```python
from build123d import *

# Parameters (mm, degrees)
SKETCH_R     = 6
PAD_DEPTH    = 9
SKETCH001_R  = 3
POCKET_DEPTH = 18.001


with BuildPart() as part:
    # Sketch → Pad (new body, symmetric)
    with BuildSketch(Plane.YZ):
        with BuildLine():
            ThreePointArc((83.569101, 625.179701), (-35.530366, 668.105579), (-91.532178, 554.56655))
            ThreePointArc((-170, 0), (-72.883506, 269.093239), (-91.532178, 554.56655))
            Line((-170, 0), (170, 0))
            ThreePointArc((170, 0), (183.382066, 320.41444), (83.569101, 625.179701))
        make_face()
        with Locations((0, 580)):
            Circle(SKETCH_R, mode=Mode.SUBTRACT)
    extrude(amount=PAD_DEPTH, both=True)

    # Sketch001 (on Face7 of Pad) → Pocket (cut, through all)
    with BuildSketch(Plane.YZ.offset(9)):
        with Locations((-53.033009, 526.966991)):
            Circle(SKETCH001_R)
        with Locations((53.033009, 526.966991)):
            Circle(SKETCH001_R)
    extrude(amount=-POCKET_DEPTH, mode=Mode.SUBTRACT)


solid = part.part
```
Work out the finished part from the listing and answer in its coordinate system (mm). Round coordinates to 2 decimals unless told otherwise and drop trailing zeros. Write each loop counter-clockwise with the first axis right and the second up, starting at its lowest first coordinate (ties: lowest second). Pieces come first, ordered by that corner, then holes. Notation, with made-up numbers: (-29.5, 3.25) -> (-21.5, 3.25) arc R15 ccw to (-21.5, 10.25) -> close; hole circle Ø2 at (2, -33.5). An arc over 180 degrees is marked (long way). Write each question's results on one line, items separated by ' | '.
1) The part is cut by section A-A (x = 0.25). Write down the section's boundary in (y, z).
Findings:
outline: (-170, 0) -> (170, 0) arc R900 ccw to (83.57, 625.18) arc R95 ccw to (-91.53, 554.57) arc R700 cw to start; hole circle Ø6 at (-53.03, 526.97); hole circle Ø12 at (0, 580); hole circle Ø6 at (53.03, 526.97)
2) The part is cut by section B-B (y = 97). Write down the section's boundary in (x, z).
Findings:
outline: (-9, 0) -> (9, 0) -> (9, 599.35) -> (-9, 599.35) -> close
3) The part is cut by section C-C (z = 175). Write down the section's boundary in (x, y).
Findings:
outline: (-9, -92.87) -> (9, -92.87) -> (9, 191.59) -> (-9, 191.59) -> close
4) Consider line 1 along Y through (x, z) = (-3.5, 580); line 2 along Z through (x, y) = (-2.75, -11); line 3 along Y through (x, z) = (-4, 568.5). Determine where each line is inside the solid, lowest interval first. Write a range as [from, to].
Findings:
line 1: y = [-95, -6], [6, 106.38] | line 2: z = [0, 674.36] | line 3: y = [-94.3, 111.68]
5) Flat-ended cylindrical pins translate along their axes: pin 1 (10 mm diameter, centred on x = 1, z = 524.5, fed in from +Y); pin 2 (5 mm diameter, centred on x = 0, z = 163.5, fed in from -Y); pin 3 (10 mm diameter, centred on x = 1.5, z = 593, fed in from +Y). Find the tip coordinate at first contact, or state that the pin passes through.
Findings:
pin 1: stops at y = 132.16 | pin 2: stops at y = -97.03 | pin 3: stops at y = 102.57
6) For a pull along Z with two mould halves and no side action, classify faces 1 (the flat face through (9, 49, 267)), 2 (the flat face through (0, -2, 0)), 3 (the cylindrical face through (-0.13, -0.78, 585.95)) as +Z half, -Z half, draft (parallel to the pull), parting line (faces both ways), or undercut.
Findings:
face 1: draft | face 2: -Z half | face 3: undercut
